Part model, mm, in its own coordinate system. A direction names the side the tool comes from. Round coordinates to 2 decimals unless told otherwise and drop trailing zeros. Write each loop counter-clockwise with the first axis right and the second up, starting at its lowest first coordinate (ties: lowest second). Pieces come first, ordered by that corner, then holes.
from build123d import *

# Parameters (mm, degrees)
F0_W     = 600
F0_H     = 850
F0_W_2   = 570
F0_H_2   = 820
F1_DEPTH = 20
F2_W     = 600
F2_H     = 850
F3_DEPTH = 5
F4_W     = 570
F4_H     = 820
F5_DEPTH = 25


with BuildPart() as f1:
    # F0 (on Front) → F1 (new body)
    with BuildSketch(Plane.XZ):
        with Locations((260.588973, 360.083479)):
            Rectangle(F0_W, F0_H)
        with Locations((260.588973, 360.083479)):
            Rectangle(F0_W_2, F0_H_2, mode=Mode.SUBTRACT)
    extrude(amount=F1_DEPTH)

    # F2 (on face) → F3 (join)
    with BuildSketch(Plane.XZ.offset(20)):
        with Locations((260.588973, 360.083479)):
            Rectangle(F2_W, F2_H)
    extrude(amount=-F3_DEPTH)

    # F4 (on face) → F5 (cut)
    with BuildSketch(Plane(origin=(0, -15, 0), x_dir=(-1, 0, 0), z_dir=(0, 1, 0))):
        with Locations((-260.588973, 360.083479)):
            Rectangle(F4_W, F4_H)
    extrude(amount=-F5_DEPTH, mode=Mode.SUBTRACT)


solid = f1.part
Q1. Saw through at A-A, the plane z = 64. Write the cut outline in (x, y).
Q2. Two-plate mould, pull along X, no slides. Class faces 1 (the flat face through (-39.411, -10, 354)), 2 (the flat face through (257, -10, 770.083)), 3 (the flat face through (560.589, -10, 354)): released by +X, released by -X, zero draft, split by the parting line, or undercut.
Q3. Tool access for faces 4 (the flat face through (259, -20, 771)), 5 (the flat face through (257, -10, -49.917)): list every direction of +Z, -Z, +X, -X, +Y, -Y with a clear straight run to the whole face (end or side of a thin tool).
Q4. Saw through at C-C, the plane y = -13.5. Write the cut outline in (x, z), and give its area (3 significant figures).
Q5. Wall check: line 1 (X direction, y = -4.5, z = 116.5); line 2 (Z direction, x = 195.5, y = -0.75). Give the ranges that are in metal, low to high.
Q6. Saw through at B-B, the plane x = 224. Write the cut outline in (y, z), and give its area (3 significant figures).
Computed:
1. outline: (-39.41, -20) - (-24.41, -20) - (-24.41, 0) - (-39.41, 0) - close; (545.59, -20) - (560.59, -20) - (560.59, 0) - (545.59, 0) - close
2. face 1: released by -X
2. face 2: undercut
2. face 3: released by +X
3. face 4: +Z, -Z, +X, -X, -Y
3. face 5: +Y, -Y
4. outline: (-39.41, -64.92) - (560.59, -64.92) - (560.59, 785.08) - (-39.41, 785.08) - close; hole (-24.41, -49.92) - (545.59, -49.92) - (545.59, 770.08) - (-24.41, 770.08) - close
4. area: 42,600 mm2
5. line 1: x = -39.41 to -24.41, 545.59 to 560.59
5. line 2: z = -64.92 to -49.92, 770.08 to 785.08
6. outline: (-20, -64.92) - (0, -64.92) - (0, -49.92) - (-20, -49.92) - close; (-20, 770.08) - (0, 770.08) - (0, 785.08) - (-20, 785.08) - close
6. area: 600 mm2
